Input: part model. Units: mm. Frame: model coordinates. Face numbers are marked on the shaded views. A direction names the side the tool comes from. Coordinates: 2 decimals unless noted, no trailing zeros. Write each loop counter-clockwise with the first axis right and the second up, starting at its lowest first coordinate (ties: lowest second). Pieces come first, ordered by that corner, then holes. Notation, with made-up numbers: (-4.75, 38.25) -> (38.25, 38.25) arc R23 ccw to (38.25, 72.25) -> close; hole circle Ø6 at (-20.5, 48). An arc over 180 degrees is marked (long way). Use one line per item in the form item = value. Start each with the question number.
(1) Ray query, line 1 along X through (y, z) = (-107.5, 5); line 2 along Z through (x, y) = (-17.5, -130); line 3 along X through (y, z) = (-135, 1.5). Return the intervals inside material, ascending.
(2) Set-up query: the marked faces 1 and 2. Return all of +Z, -Z, +X, -X, +Y, -Y with unobstructed straight access to the full face (end or side cutting, diameter ignored); none if empty.
(3) Cut plane B-B on x = -3. Return the cut outline in (y, z), plus the area to 3 significant figures.
(4) First-contact query: pin 1 (1.5 mm diameter, centred on x = -8, y = -56, fed in from +Z); pin 2 (3 mm diameter, centred on y = -51.5, z = 4.5, fed in from +X); pin 3 (1.6 mm diameter, centred on x = -27.5, y = -144, fed in from -Z); pin 4 (2 mm diameter, centred on x = -18, z = 3, fed in from -Y). Flat tips, straight axial feed; report the tip coordinate or a pass-through.
(5) Cut plane A-A on y = -124.5. Return the cut outline in (x, z), plus the area to 3 significant figures.
```python
from build123d import *

# Parameters (mm, degrees)
F1_DEPTH = 200


with BuildPart() as f1:
    # F0 (on Front) → F1 (new body)
    with BuildSketch(Plane.XZ):
        with BuildLine():
            Line((-23.4, 0), (0, 0))
            ThreePointArc((0, 0), (1.272792, 0.527208), (1.8, 1.8))
            Line((1.8, 1.8), (1.8, 5.7))
            ThreePointArc((1.8, 5.7), (2.034315, 6.265685), (2.6, 6.5))
            Line((2.6, 6.5), (5.7996, 6.5))
            Line((5.7996, 6.5), (5.8004, 7.5))
            Line((5.8004, 7.5), (2.6, 7.5))
            ThreePointArc((2.6, 7.5), (1.327208, 6.972792), (0.8, 5.7))
            Line((0.8, 5.7), (0.8, 1.8))
            ThreePointArc((0.8, 1.8), (0.565685, 1.234315), (0, 1))
            Line((0, 1), (-23.4, 1))
            ThreePointArc((-23.4, 1), (-23.965685, 1.234315), (-24.2, 1.8))
            Line((-24.2, 1.8), (-24.2, 5.7))
            ThreePointArc((-24.2, 5.7), (-24.727208, 6.972792), (-26, 7.5))
            Line((-26, 7.5), (-29.2004, 7.5))
            Line((-29.2004, 7.5), (-29.2004, 6.5))
            Line((-29.2004, 6.5), (-26, 6.5))
            ThreePointArc((-26, 6.5), (-25.434315, 6.265685), (-25.2, 5.7))
            Line((-25.2, 5.7), (-25.2, 1.8))
            ThreePointArc((-25.2, 1.8), (-24.672792, 0.527208), (-23.4, 0))
        make_face()
    extrude(amount=F1_DEPTH)


solid = f1.part
```
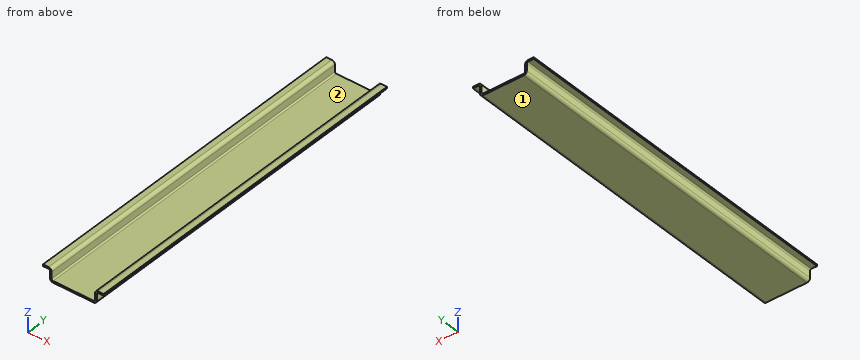
Values:
q1.line_1 = -25.2 to -24.2, 0.8 to 1.8
q1.line_2 = 0 to 1
q1.line_3 = -25.17 to -24.14, 0.74 to 1.77
q2.face_1 = -Z, +X, -X, +Y, -Y
q2.face_2 = +Z, +Y, -Y
q3.outline = (-200, 0) -> (0, 0) -> (0, 1) -> (-200, 1) -> close
q3.area = 200 mm2
q4.pin_1 = 1
q4.pin_2 = 1.86
q4.pin_3 = 6.5
q4.pin_4 = through
q5.outline = (-29.2, 6.5) -> (-26, 6.5) arc R0.8 cw to (-25.2, 5.7) -> (-25.2, 1.8) arc R1.8 ccw to (-23.4, 0) -> (0, 0) arc R1.8 ccw to (1.8, 1.8) -> (1.8, 5.7) arc R0.8 cw to (2.6, 6.5) -> (5.8, 6.5) -> (5.8, 7.5) -> (2.6, 7.5) arc R1.8 ccw to (0.8, 5.7) -> (0.8, 1.8) arc R0.8 cw to (0, 1) -> (-23.4, 1) arc R0.8 cw to (-24.2, 1.8) -> (-24.2, 5.7) arc R1.8 ccw to (-26, 7.5) -> (-29.2, 7.5) -> close
q5.area = 45.8 mm2
